```python
from build123d import *

# Parameters (mm, degrees)
BASE_FLANGE2_DEPTH = 20
FILLET1_R          = 7
SKETCH17_R         = 3
CUT_EXTRUDE1_DEPTH = 51.329697794


# Sheet-metal steps are written as plain solids
with BuildPart() as part:
    # Sketch12 → Base-Flange2 (new body)
    with BuildSketch(Plane(origin=(0, 0, 0), x_dir=(1, 0, 0), z_dir=(0, 1, 0))):
        with BuildLine():
            Line((-31.764, 0), (-19.5006, 0))
            ThreePointArc((-19.5006, 0), (-17.565531583, 0.801531583), (-16.764, 2.7366))
            Line((-16.764, 2.7366), (-16.764, 16.764))
            ThreePointArc((-16.764, 16.764), (0, 33.528), (16.764, 16.764))
            Line((16.764, 16.764), (16.764, 2.7366))
            ThreePointArc((16.764, 2.7366), (17.565531583, 0.801531583), (19.5006, 0))
            Line((19.5006, 0), (31.764, 0))
            Line((31.764, 0), (31.764, 2))
            Line((31.764, 2), (19.5006, 2))
            ThreePointArc((19.5006, 2), (18.979745145, 2.215745145), (18.764, 2.7366))
            Line((18.764, 2.7366), (18.764, 16.764))
            ThreePointArc((18.764, 16.764), (0, 35.528), (-18.764, 16.764))
            Line((-18.764, 16.764), (-18.764, 2.7366))
            ThreePointArc((-18.764, 2.7366), (-18.979745145, 2.215745145), (-19.5006, 2))
            Line((-19.5006, 2), (-31.764, 2))
            Line((-31.764, 2), (-31.764, 0))
        make_face()
    extrude(amount=BASE_FLANGE2_DEPTH)

    # Fillet1
    fillet1_edges = [part.edges().sort_by_distance(p)[0] for p in [
        (-31.764, 0, -1),
        (31.764, 0, -1),
        (-31.764, 20, -1),
        (31.764, 20, -1),
    ]]
    fillet(fillet1_edges, radius=FILLET1_R)

    # Sketch17 → Cut-Extrude1 (cut, through all)
    with BuildSketch(Plane(origin=(0, 0, -2), x_dir=(-1, 0, 0), z_dir=(0, 0, -1))):
        with Locations((24.764, 10)):
            Circle(SKETCH17_R)
    cut_extrude1 = extrude(amount=-CUT_EXTRUDE1_DEPTH, mode=Mode.SUBTRACT)

    # Mirror1: Cut-Extrude1 across plane
    add(cut_extrude1.mirror(Plane(origin=(0, 0, 0), x_dir=(0, 0, 1), z_dir=(1, 0, 0))), mode=Mode.SUBTRACT)


solid = part.part
```
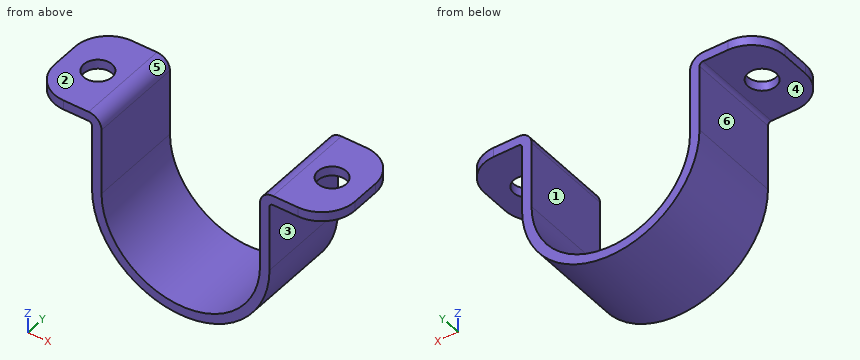
Read the model definition and answer for the solid it produces. Units are mm, in the model's axes. Face numbers are marked on the shaded views. A direction names the side the tool comes from. Round coordinates to 2 decimals unless told otherwise and drop trailing zeros. Write each loop counter-clockwise with the first axis right and the second up, starting at its lowest first coordinate (ties: lowest second). Pieces come first, ordered by that corner, then holes. Notation, with made-up numbers: (53.5, 78) -> (97.5, 78) arc R5 cw to (97.5, 83) -> close; hole circle Ø6 at (75.25, 19.5). An arc over 180 degrees is marked (long way). Answer in a Markdown table with one row per item. Add a question column.
1) Find section A-A, the plane y = 10. Determine the outline of the cut face in (x, z).
2) Which of the six approach directions +Z, -Z, +X, -X, +Y, -Y give full straight-line access (tool end or side, diameter ignored) to the marked faces 1, 2 and 3?
3) Determine the mould class of the marked faces 4, 5 and 6 for opening direction X: pulls with the +X half, pulls with the -X half, needs draft (parallel to the pull), parting line crosses it, or undercut.
4) Find section D-D, the plane y = 15.25. Determine the outline of the cut face in (x, z), and give its area (3 significant figures).
5) Find section B-B, the plane z = -5. Determine the outline of the cut face in (x, y), and give its area (3 significant figures).
6) Given P1, Ø3.5, axis at x = -23.5, y = 15, coming from the -Z side; P2, Ø3.5, axis at x = -24.764, y = 10, coming from the +Z side; P3, Ø4, axis at y = 13, z = -18, coming from the +X side; P4, Ø8, axis at x = -8, y = 2.5, coming from the +Z side, each flat-ended and moving along its own axis, determine where each tip first touches the part or whether it passes through.
7) Consider line 1 (X direction, y = 4, z = -9); line 2 (X direction, y = 16.5, z = -21); line 3 (Z direction, x = 0.5, y = 11). Determine where each line is inside the solid, lowest interval first.
8) Find section C-C, the plane x = 25.5. Determine the outline of the cut face in (y, z), and give its area (3 significant figures).
Findings below:
| question | item | result |
|---|---|---|
| 1 | outline | (-31.76, -2) -> (-27.76, -2) -> (-27.76, 0) -> (-31.76, 0) -> close; (-21.76, -2) -> (-19.5, -2) arc R0.74 cw to (-18.76, -2.74) -> (-18.76, -16.76) arc R18.76 ccw to (18.76, -16.76) -> (18.76, -2.74) arc R0.74 cw to (19.5, -2) -> (21.76, -2) -> (21.76, 0) -> (19.5, 0) arc R2.74 ccw to (16.76, -2.74) -> (16.76, -16.76) arc R16.76 cw to (-16.76, -16.76) -> (-16.76, -2.74) arc R2.74 ccw to (-19.5, 0) -> (-21.76, 0) -> close; (27.76, -2) -> (31.76, -2) -> (31.76, 0) -> (27.76, 0) -> close |
| 2 | face 1 | +Z, +Y, -Y |
| 2 | face 2 | +Z, +X, -X, +Y, -Y |
| 2 | face 3 | -Z, +X, +Y, -Y |
| 3 | face 4 | needs draft |
| 3 | face 5 | undercut |
| 3 | face 6 | pulls with the -X half |
| 4 | outline | (-31.39, -2) -> (-19.5, -2) arc R0.74 cw to (-18.76, -2.74) -> (-18.76, -16.76) arc R18.76 ccw to (18.76, -16.76) -> (18.76, -2.74) arc R0.74 cw to (19.5, -2) -> (31.39, -2) -> (31.39, 0) -> (19.5, 0) arc R2.74 ccw to (16.76, -2.74) -> (16.76, -16.76) arc R16.76 cw to (-16.76, -16.76) -> (-16.76, -2.74) arc R2.74 ccw to (-19.5, 0) -> (-31.39, 0) -> close |
| 4 | area | 226 mm² |
| 5 | outline | (-18.76, 0) -> (-16.76, 0) -> (-16.76, 20) -> (-18.76, 20) -> close; (16.76, 0) -> (18.76, 0) -> (18.76, 20) -> (16.76, 20) -> close |
| 5 | area | 80.0 mm² |
| 6 | P1 | z = -2 |
| 6 | P2 | through |
| 6 | P3 | x = 18.76 |
| 6 | P4 | z = -28.47 |
| 7 | line 1 | -18.76 to -16.76, 16.76 to 18.76 |
| 7 | line 2 | -18.28 to -16.22, 16.22 to 18.28 |
| 7 | line 3 | -35.52 to -33.52 |
| 8 | outline | (0.04, -2) -> (7.09, -2) -> (7.09, 0) -> (0.04, 0) -> close; (12.91, -2) -> (19.96, -2) -> (19.96, 0) -> (12.91, 0) -> close |
| 8 | area | 28.2 mm² |
